Here's how the part is built. I have some questions about the finished solid (model axes, mm). A direction names the side the tool comes from. Round coordinates to 2 decimals unless told otherwise and drop trailing zeros. Loops run counter-clockwise (first coordinate to the right, second up) from the corner with the lowest first, then second, coordinate; pieces in that order, holes last. Notation, with made-up numbers: M 21,64.25 L 27,64.25 A18 cw 27,85.25 Z; hole C 8,33 d11. An arc over 180 degrees is marked long. Use a Markdown table: item, result.
from build123d import *

# Parameters (mm, degrees)
F0_R      = 4.5
F1_DEPTH  = 19
F2_DEPTH  = 57.3
F3_R      = 5.5
F4_DEPTH  = 1
F6_R      = 1.5
F7_DEPTH  = 10
F8_R      = 0.9
F9_DEPTH  = 10
F10_R     = 4.5
F12_DEPTH = 3.5
F11_R     = 5.5
F11_R_2   = 4.5
F13_DEPTH = 1


# Not quite as in the source:
# - a fillet or chamfer that OpenCascade refuses, or shapes differently, is made with other operations: its cross-section is extruded or revolved along the edge and cut away or added


with BuildPart() as f1:
    # F0 (on Front) → F1 (new body)
    with BuildSketch(Plane.XZ):
        Circle(F0_R)
    extrude(amount=F1_DEPTH)

    # F2 (add): a face of the model
    f2_faces = [f1.faces().sort_by_distance(p)[0] for p in [
        (0, 0, 0),
    ]]
    extrude(f2_faces, amount=F2_DEPTH)

    # F3 (on Front) → F4 (join)
    with BuildSketch(Plane.XZ):
        Circle(F3_R)
    extrude(amount=-F4_DEPTH)

    # F5: fillet of radius 5 on 2 edges, made by hand

    # F5_s1 → F5_t2 (revolve)
    with BuildSketch(Plane.XY):
        with BuildLine():
            ThreePointArc((4.5, -3), (4.7565835097, -1.4188611699), (5.5, 0))
            Line((5.5, 0), (4.5, 0))
            Line((4.5, 0), (4.5, -3))
        make_face()
    revolve(axis=Axis((0, 0, 0), (0, -1, 0)))

    # F5_s3 → F5_t4 (revolve)
    with BuildSketch(Plane.XY):
        with BuildLine():
            ThreePointArc((5.5, 1), (4.7565835097, 2.4188611699), (4.5, 4))
            Line((4.5, 4), (4.5, 1))
            Line((4.5, 1), (5.5, 1))
        make_face()
    revolve(axis=Axis((0, 1, 0), (0, -1, 0)))

    # F6 (on face) → F7 (cut)
    with BuildSketch(Plane.XZ.offset(19)):
        Circle(F6_R)
    extrude(amount=-F7_DEPTH, mode=Mode.SUBTRACT)

    # F8 (on face) → F9 (join)
    with BuildSketch(Plane.XZ.offset(19)):
        with Locations((-3, 0)):
            Circle(F8_R)
        with Locations((0, -3)):
            Circle(F8_R)
        with Locations((3, 0)):
            Circle(F8_R)
        with Locations((0, 3)):
            Circle(F8_R)
    extrude(amount=F9_DEPTH)

    # F10 (on face) → F12 (join)
    with BuildSketch(Plane(origin=(0, 57.3, 0), x_dir=(-1, 0, 0), z_dir=(0, 1, 0))):
        Circle(F10_R)
    extrude(amount=F12_DEPTH)

    # F11 (on face) → F13 (join)
    with BuildSketch(Plane(origin=(0, 57.3, 0), x_dir=(-1, 0, 0), z_dir=(0, 1, 0))):
        Circle(F11_R)
        Circle(F11_R_2, mode=Mode.SUBTRACT)
    extrude(amount=-F13_DEPTH)

    # F14: fillet of radius 5 on 1 edges, made by hand

    # F14_s1 → F14_t2 (revolve)
    with BuildSketch(Plane.XY):
        with BuildLine():
            ThreePointArc((4.5, 53.3), (4.7565835097, 54.8811388301), (5.5, 56.3))
            Line((5.5, 56.3), (4.5, 56.3))
            Line((4.5, 56.3), (4.5, 53.3))
        make_face()
    revolve(axis=Axis((0, 56.3, 0), (0, -1, 0)))


solid = f1.part
1. I need wall thicknesses on probe 1 along Z at (x, y) = (0, -15); probe 2 along Y at (x, z) = (-2.5, -2.25); probe 3 along Z at (x, y) = (0.25, -3). Which ranges of each line are inside material? Lowest first, please. Write a range as from..to.
Answer sheet:
| item | result |
|---|---|
| probe 1 | -4.5..-1.5, 1.5..4.5 |
| probe 2 | -19..60.8 |
| probe 3 | -4.49..4.49 |
2. We'd pull the mould along X, two halves only. Please class faces 5 (the face through (0, 60.8, 0)), 6 (the face through (-1.5, -14.07, 0.07)), 7 (the face through (1.19, 56.81, -5.37)): +X half, -X half, draft (parallel to the pull), parting line (faces both ways), or undercut.
Answer sheet:
| item | result |
|---|---|
| face 5 | draft |
| face 6 | undercut |
| face 7 | parting line |
3. Imagine slicing it at B-B, the plane y = 40. Write out the boundary of the cut face in (x, z), then the cut area to 3 significant figures.
Answer sheet:
| item | result |
|---|---|
| outline | C 0,0 d9 |
| area | 63.6 mm2 |
4. Which directions (+Z, -Z, +X, -X, +Y, -Y) give clear straight access to the entire face, cutting with the end or side of a thin tool? Please do faces 1 (the face through (-2.14, -23.93, 0.27)), 2 (the face through (3, -29, 0)), 3 (the face through (-0.59, 28.3, 4.46)), 4 (the face through (5, 57.3, 0)).
Answer sheet:
| item | result |
|---|---|
| face 1 | -Y |
| face 2 | +Z, -Z, +X, -X, -Y |
| face 3 | none |
| face 4 | +Y |
5. For pin 1 Ø1.5 at (x, z) = (-0.5, 0.5) entering from -Y; pin 2 Ø4 at (y, z) = (51.5, -1.5) entering from +X; pin 3 Ø1.5 at (x, y) = (0.5, -14.5) entering from -Z, each with a flat end and sliding along its axis, tell me the tip position at first contact or that it passes through.
Answer sheet:
| item | result |
|---|---|
| pin 1 | y = -9 |
| pin 2 | x = 4.5 |
| pin 3 | z = -4.5 |
